Part model, mm, in its own coordinate system. Face numbers are marked on the shaded views. A direction names the side the tool comes from. Round coordinates to 2 decimals unless told otherwise and drop trailing zeros. Loops run counter-clockwise (first coordinate to the right, second up) from the corner with the lowest first, then second, coordinate; pieces in that order, holes last. Notation, with made-up numbers: M -20.75,55.25 L -3.75,55.25 A23 ccw -3.75,81.25 Z; hole C 70,18 d1. An arc over 180 degrees is marked long. Put each result on its own line as item: value. Start each with the question number.
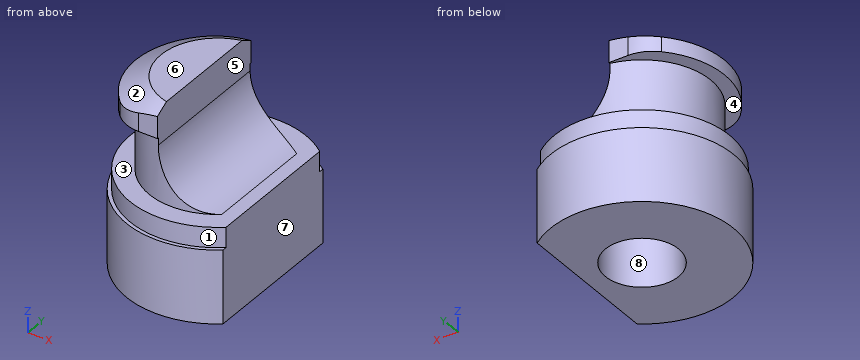
```python
from build123d import *
from OCP.BRepFilletAPI import BRepFilletAPI_MakeChamfer

# Parameters (mm, degrees)
SKETCH1_R               = 2.4
BOSS_EXTRUDE1_DEPTH     = 0.55
SKETCH2_R               = 1.875
BOSS_EXTRUDE2_DEPTH     = 1.7
SKETCH3_R               = 2.5
BOSS_EXTRUDE3_DEPTH     = 2
SKETCH4_R               = 2.25
BOSS_EXTRUDE4_DEPTH     = 0.8
CUT_EXTRUDE1_REACH      = 8.165
SKETCH5_W               = 0.75
SKETCH5_H               = 6.07376998
CHAMFER1_SIZE           = 0.4
CHAMFER1_SIZE2          = 0.692820323
SKETCH6_W               = 6.999273813
SKETCH6_H               = 5.334981493
SKETCH6_W_2             = 6.558585844
SKETCH6_H_2             = 3.75
CUT_EXTRUDE3_DEPTH      = 2
FILLET2_R               = 1
SKETCH7_R               = 1
CUT_EXTRUDE4_DEPTH      = 2
CUT_EXTRUDE5_DEPTH      = 3
CUT_EXTRUDE5_DEPTH_BACK = 10
SKETCH9_W               = 3.309409713
SKETCH9_H               = 2.920914296
FILLET3_R               = 1.5
SKETCH10_W              = 2.950077704
SKETCH10_H              = 6.497759574
CUT_EXTRUDE6_DEPTH      = 10


with BuildPart() as part:
    # Sketch1 → Boss-Extrude1 (new body)
    with BuildSketch(Plane.XY):
        Circle(SKETCH1_R)
    extrude(amount=BOSS_EXTRUDE1_DEPTH)

    # Sketch2 → Boss-Extrude2 (add)
    with BuildSketch(Plane.XY.offset(0.55)):
        Circle(SKETCH2_R)
    extrude(amount=BOSS_EXTRUDE2_DEPTH)

    # Sketch3 → Boss-Extrude3 (add)
    with BuildSketch(Plane(origin=(0, 0, 0), x_dir=(-1, 0, 0), z_dir=(0, 0, -1))):
        Circle(SKETCH3_R)
    extrude(amount=BOSS_EXTRUDE3_DEPTH)

    # Sketch4 → Boss-Extrude4 (add)
    with BuildSketch(Plane.XY.offset(2.25)):
        Circle(SKETCH4_R)
    extrude(amount=BOSS_EXTRUDE4_DEPTH)

    # Cut-Extrude1: up to this face of the body (flat: up to its plane)
    cut_extrude1_end = Plane(part.part.faces().sort_by_distance((-2.332117749, 0, 0.55))[0])
    # Sketch5 → Cut-Extrude1 (cut, up to the picked face)
    with BuildSketch(Plane.XY.offset(3.05), mode=Mode.PRIVATE) as cut_extrude1_sk1:
        Rectangle(SKETCH5_W, SKETCH5_H)
    cut_extrude1_tool1 = split(extrude(cut_extrude1_sk1.sketch, amount=-CUT_EXTRUDE1_REACH, mode=Mode.PRIVATE), bisect_by=cut_extrude1_end, keep=Keep.BOTH, mode=Mode.PRIVATE)
    add(cut_extrude1_tool1.solids().sort_by(Axis((0, 0, 3.05), (0, 0, -1)))[0], mode=Mode.SUBTRACT)

    # Chamfer1: one chamfer whose edges measure the first distance from different faces: ONE call of the kernel's chamfer builder (chamfer() names one face for all edges)
    chamfer1_edges_1 = [part.edges().sort_by_distance(p)[0] for p in [
        (-2.25, 0, 3.05),
    ]]
    chamfer1_side_1 = [part.faces().sort_by_distance(p)[0] for p in [
        (-2.25, 0, 2.65),
    ]]
    chamfer1_edges_2 = [part.edges().sort_by_distance(p)[0] for p in [
        (2.25, 0, 3.05),
    ]]
    chamfer1_side_2 = [part.faces().sort_by_distance(p)[0] for p in [
        (2.25, 0, 2.65),
    ]]
    chamfer1 = BRepFilletAPI_MakeChamfer(part.part.solid().wrapped)
    for e in chamfer1_edges_1:
        chamfer1.Add(CHAMFER1_SIZE, CHAMFER1_SIZE2, e.wrapped, chamfer1_side_1[0].wrapped)  # the first distance lies on this face
    for e in chamfer1_edges_2:
        chamfer1.Add(CHAMFER1_SIZE, CHAMFER1_SIZE2, e.wrapped, chamfer1_side_2[0].wrapped)  # the first distance lies on this face
    add(Compound.cast(chamfer1.Shape()), mode=Mode.REPLACE)

    # Sketch6 → Cut-Extrude3 (cut)
    with BuildSketch(Plane.XY.offset(3.05)):
        with Locations((0.047792, -0.043471688)):
            Rectangle(SKETCH6_W, SKETCH6_H)
        Rectangle(SKETCH6_W_2, SKETCH6_H_2, mode=Mode.SUBTRACT)
    extrude(amount=-CUT_EXTRUDE3_DEPTH, mode=Mode.SUBTRACT)

    # Fillet2
    fillet2_edges = [part.edges().sort_by_distance(p)[0] for p in [
        (-1.243734296, 1.875, 2.45),
        (1.243734296, 1.875, 2.45),
        (-1.243734296, -1.875, 2.45),
        (1.243734296, -1.875, 2.45),
    ]]
    fillet(fillet2_edges, radius=FILLET2_R)

    # Sketch7 → Cut-Extrude4 (cut)
    with BuildSketch(Plane(origin=(0, 0, -2), x_dir=(-1, 0, 0), z_dir=(0, 0, -1))):
        Circle(SKETCH7_R)
    extrude(amount=-CUT_EXTRUDE4_DEPTH, mode=Mode.SUBTRACT)

    # Sketch9 → Cut-Extrude5 (cut, two sides: drawn at the far end of the back side and taken through both)
    with BuildSketch(Plane(origin=(0, 0, 0), x_dir=(1, 0, 0), z_dir=(0, 1, 0)).offset(-CUT_EXTRUDE5_DEPTH_BACK)):
        with Locations((1.654704857, -2.010457148)):
            Rectangle(SKETCH9_W, SKETCH9_H)
    extrude(amount=CUT_EXTRUDE5_DEPTH + CUT_EXTRUDE5_DEPTH_BACK, mode=Mode.SUBTRACT)

    # Fillet3
    fillet3_edges = [part.edges().sort_by_distance(p)[0] for p in [
        (-0.375, 0, 0.55),
    ]]
    fillet(fillet3_edges, radius=FILLET3_R)

    # Sketch10 → Cut-Extrude6 (cut)
    with BuildSketch(Plane.XY.offset(0.55)):
        with Locations((2.975038852, 0.087286089)):
            Rectangle(SKETCH10_W, SKETCH10_H)
    extrude(amount=-CUT_EXTRUDE6_DEPTH, mode=Mode.SUBTRACT)


solid = part.part
```
1. Drop flat-ended pins along their axis: pin 1 (0.8 mm diameter, centred on y = -0.5, z = 2.5, fed in from +X) (3 decimals); pin 2 (1.6 mm diameter, centred on x = 0, y = -0.5, fed in from -Z); pin 3 (1.5 mm diameter, centred on y = -1.5, z = 1, fed in from -X). Give the stop position or say it passes through.
2. Cut at B-B, the plane x = 0.2. Give the cut face in (y, z).
3. Wall check: L1, parallel to Y at x = 0, z = -1.15; L2, parallel to Y at x = -0.8, z = -1.45; L3, parallel to Z at x = 0.35, y = 1.9. Give the ranges that are in metal, low to high.
4. Mould opens along X. For the marked faces 6, 7 and 8 say: released by +X, released by -X, zero draft, split by the parting line, or undercut.
5. Which spindle directions (+Z, -Z, +X, -X, +Y, -Y) get a long thin tool onto all of the face, cutting with end or side? Do the marked faces 1, 2, 3, 4 and 5. Say none if no direction does.
6. Cut at C-C, the plane z = -1. Give the cut face in (x, y), and give its area (3 significant figures).
7. Cut at A-A, the plane y = 0. Give the cut face in (x, z) (3 decimals).
Results list:
1. pin 1: stops at x = -0.375
1. pin 2: stops at z = -2
1. pin 3: stops at x = -2.22
2. outline: M -2.49,-2 L -0.98,-2 L -0.98,0 L 0.98,0 L 0.98,-2 L 2.49,-2 L 2.49,0 L 2.39,0 L 2.39,0.55 L 1.86,0.55 L 1.86,0.87 L -1.86,0.87 L -1.86,0.55 L -2.39,0.55 L -2.39,0 L -2.49,0 Z
3. L1: y = -2.5 to -1, 1 to 2.5
3. L2: y = -2.37 to -0.6, 0.6 to 2.37
3. L3: z = -2 to 0.55
4. face 6: zero draft
4. face 7: released by +X
4. face 8: undercut
5. face 1: +Z
5. face 2: +Z, -X
5. face 3: none
5. face 4: -X
5. face 5: +Z, +X, +Y, -Y
6. outline: M 1.5,-2 L 1.5,2 A2.5 ccw long Z; hole C 0,0 d2
6. area: 13.7 mm^2
7. outline: M -2.5,-2 L -1,-2 L -1,0 L 1,0 L 1,-2 L 1.5,-2 L 1.5,0.55 L 1.125,0.55 A1.5 cw -0.375,2.05 L -0.375,3.05 L -1.557,3.05 L -2.25,2.65 L -2.25,2.25 L -1.875,2.25 L -1.875,0.55 L -2.4,0.55 L -2.4,0 L -2.5,0 Z
